Geometry check sheet. Reference: the model listing, model coordinates, mm. Face numbers are marked on the shaded views. Coordinates: 2 decimals unless noted, no trailing zeros. Write each loop counter-clockwise with the first axis right and the second up, starting at its lowest first coordinate (ties: lowest second). Pieces come first, ordered by that corner, then holes. Notation, with made-up numbers: (-38, 5.25) -> (-25, 5.25) arc R20 cw to (-25, 9.25) -> close; hole circle Ø8 at (50, 29). An arc over 180 degrees is marked (long way). Use a Markdown table: item, result.
```python
from build123d import *

# Parameters (mm, degrees)
BOSS_EXTRUDE1_DEPTH = 5
SKETCH1_3_R         = 1.5
CUT_EXTRUDE1_DEPTH  = 3
FILLET1_R           = 1
FILLET2_R           = 0.5


with BuildPart() as part:
    # Sketch1 → Boss-Extrude1 (new body)
    with BuildSketch(Plane(origin=(0, 0, 0), x_dir=(1, 0, 0), z_dir=(0, 1, 0))):
        with BuildLine():
            Line((0.5, 0.643681577), (0.5, 13))
            Line((0.5, 13), (20.5, 13))
            Line((20.5, 13), (20.5, 0.643681577))
            ThreePointArc((20.5, 0.643681577), (10.5, 0), (0.5, 0.643681577))
        make_face()
    extrude(amount=BOSS_EXTRUDE1_DEPTH)

    # Sketch1_3 → Cut-Extrude1 (cut)
    with BuildSketch(Plane(origin=(0, 0, 0), x_dir=(1, 0, 0), z_dir=(0, 1, 0))):
        with Locations(Location((5.5, 9, 0), (0, 0, 270))):
            Circle(SKETCH1_3_R)
        with Locations(Location((15.5, 9, 0), (0, 0, 270))):
            Circle(SKETCH1_3_R)
    extrude(amount=CUT_EXTRUDE1_DEPTH, mode=Mode.SUBTRACT)

    # Fillet1
    fillet1_edges = [part.edges().sort_by_distance(p)[0] for p in [
        (0.5, 2.5, -0.643681577),
        (20.5, 2.5, -0.643681577),
        (20.5, 2.5, -13),
        (0.5, 2.5, -13),
    ]]
    fillet(fillet1_edges, radius=FILLET1_R)

    # Fillet2
    fillet2_edges = [part.edges().sort_by_distance(p)[0] for p in [
        (10.5, 0, -13),
        (10.5, 5, -13),
        (0.5, 0, -6.763891411),
        (20.5, 0, -6.763891411),
        (10.5, 0, 0),
        (0.752710526, 0, -0.863284184),
        (20.247289474, 0, -0.863284184),
        (0.792893219, 0, -12.707106781),
        (20.207106781, 0, -12.707106781),
        (20.5, 5, -6.763891411),
        (0.5, 5, -6.763891411),
        (10.5, 5, 0),
        (0.752710526, 5, -0.863284184),
        (20.247289474, 5, -0.863284184),
        (0.792893219, 5, -12.707106781),
        (20.207106781, 5, -12.707106781),
    ]]
    fillet(fillet2_edges, radius=FILLET2_R)


solid = part.part
```
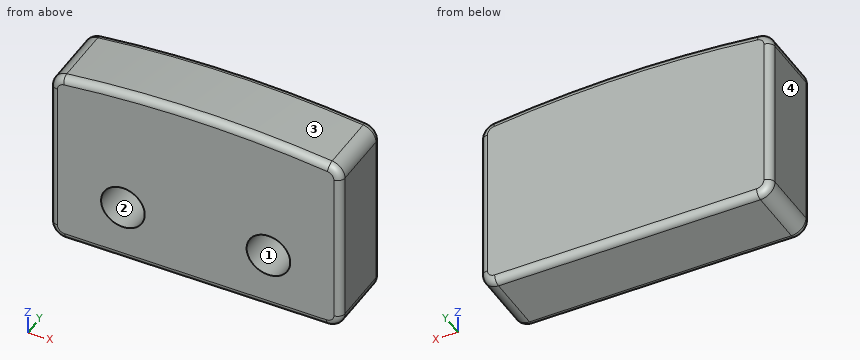
Item 1: Section check A-A on y = 2.8. Record the boundary of the cut face in (x, z), then the cut area to 3 significant figures.
Answer block:
| item | result |
|---|---|
| outline | (0.5, -12) arc R1 ccw to (1.5, -13) -> (19.5, -13) arc R1 ccw to (20.5, -12) -> (20.5, -1.53) arc R1 ccw to (19.62, -0.53) arc R78 ccw to (1.38, -0.53) arc R1 ccw to (0.5, -1.53) -> close; hole circle Ø3 at (5.5, -9); hole circle Ø3 at (15.5, -9) |
| area | 241 mm^2 |
Item 2: Thickness scan on L1, parallel to X at y = 1.6, z = -9; L2, parallel to Z at x = 6.5, y = 0.95; L3, parallel to X at y = 0.55, z = -10.25. Record the ranges inside material, lowest first. Write a range as [from, to].
Answer block:
| item | result |
|---|---|
| L1 | x = [0.5, 4], [7, 14], [17, 20.5] |
| L2 | z = [-13, -10.12], [-7.88, -0.1] |
| L3 | x = [0.5, 4.67], [6.33, 14.67], [16.33, 20.5] |
Item 3: Mould release check, pull along Z, two halves, no side actions. Record for the marked faces 1, 2, 3 and 4: +Z half, -Z half, draft (parallel to the pull), parting line (faces both ways), or undercut.
Answer block:
| item | result |
|---|---|
| face 1 | undercut |
| face 2 | undercut |
| face 3 | +Z half |
| face 4 | draft |
Item 4: Section check B-B on z = -9. Record the boundary of the cut face in (x, y).
Answer block:
| item | result |
|---|---|
| outline | (0.5, 0.5) arc R0.5 ccw to (1, 0) -> (4, 0) -> (4, 3) -> (7, 3) -> (7, 0) -> (14, 0) -> (14, 3) -> (17, 3) -> (17, 0) -> (20, 0) arc R0.5 ccw to (20.5, 0.5) -> (20.5, 4.5) arc R0.5 ccw to (20, 5) -> (1, 5) arc R0.5 ccw to (0.5, 4.5) -> close |
